Check sheet for the drawn part. Datum: minimum x, y, z corner. Units: mm. A direction names the side the tool comes from. Coordinates: 2 decimals unless noted, no trailing zeros. Order: outer loops, then holes, each group sorted by start corner. A loop starts at its lowest first (then second) coordinate and runs counter-clockwise, first axis right, second up.
1. Cross-section at D-D (y = 3.5). Enter the section's corners in (x, z), then the cut area to 3 significant figures.
2. Set-up check for the marked faces 1 and 2: record each of +Z, -Z, +X, -X, +Y, -Y from which the full face is reachable in a straight line by a thin tool's end or side.
3. Gauge pin test, flat ends, axial feed: pin 1 Ø4 at (x, y) = (9, 3) entering from +Z; pin 2 Ø2 at (y, z) = (7.5, 9) entering from -X; pin 3 Ø1 at (x, z) = (7.5, 14) entering from -Y; pin 4 Ø2 at (y, z) = (11, 12) entering from +X. Record the tip position at first contact, or that the pin passes through.
4. Draft check along Y on the marked faces 3, 4 and 5. Enter one of: released by +Y, released by -Y, zero draft, split by the parting line, or undercut.
5. Cross-section at A-A (z = 8). Enter the section's corners in (x, y).
6. Thickness scan on line 1 (X direction, y = 8, z = 9.25); line 2 (X direction, y = 8, z = 5); line 3 (Y direction, x = 5, z = 8). Record the ranges inside material, lowest first.
7. Cross-section at B-B (y = 7.75). Enter the section's corners in (x, z), then the cut area to 3 significant figures.
8. Cross-section at C-C (x = 5.5). Enter the section's corners in (y, z), then the cut area to 3 significant figures.
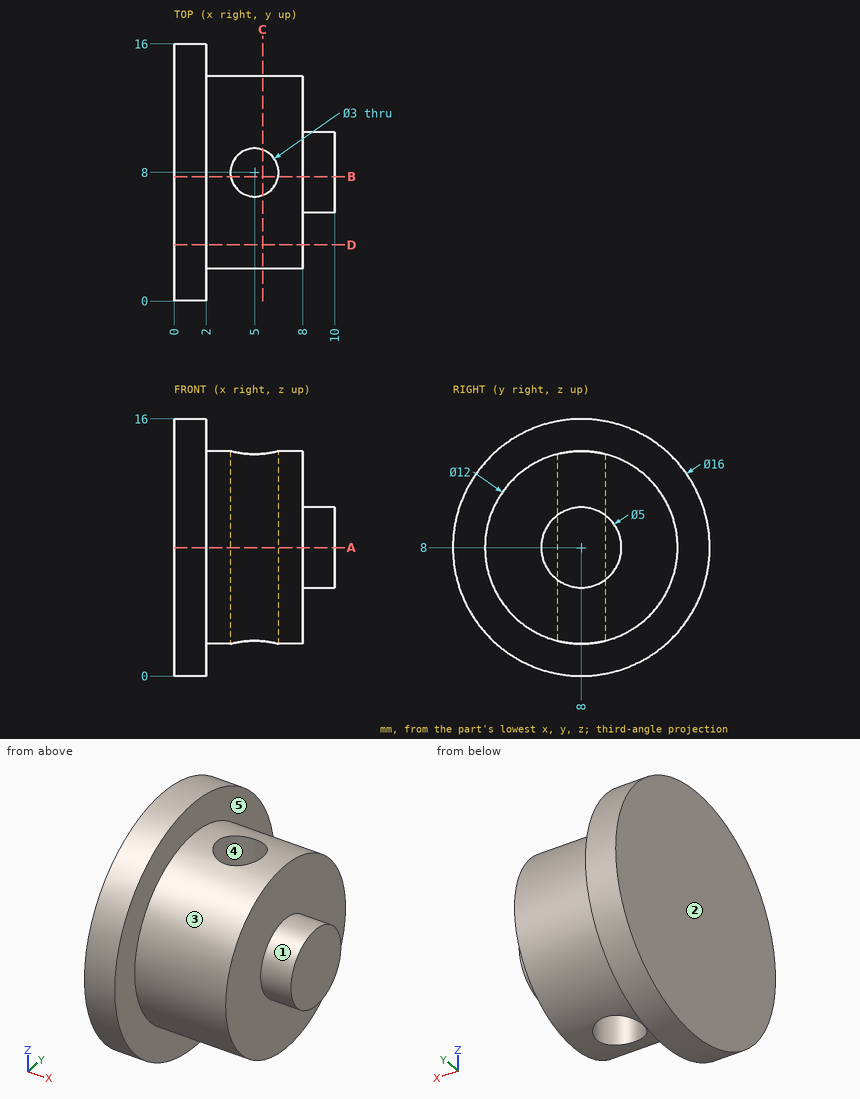
Data:
1. outline: (0, 1.39) - (2, 1.39) - (2, 4.03) - (8, 4.03) - (8, 11.97) - (2, 11.97) - (2, 14.61) - (0, 14.61) - close
1. area: 74.1 mm2
2. face 1: +X
2. face 2: +Z, -Z, -X, +Y, -Y
3. pin 1: stops at z = 13.03
3. pin 2: stops at x = 0
3. pin 3: stops at y = 5.6
3. pin 4: stops at x = 8
4. face 3: split by the parting line
4. face 4: undercut
4. face 5: zero draft
5. outline: (0, 0) - (2, 0) - (2, 2) - (8, 2) - (8, 5.5) - (10, 5.5) - (10, 10.5) - (8, 10.5) - (8, 14) - (2, 14) - (2, 16) - (0, 16) - close; hole circle Ø3 at (5, 8)
6. line 1: x = 0 to 3.5, 6.5 to 10
6. line 2: x = 0 to 3.5, 6.5 to 8
6. line 3: y = 2 to 6.5, 9.5 to 14
7. outline: (0, 0) - (2, 0) - (2, 2.01) - (3.52, 2.01) - (3.52, 13.99) - (2, 13.99) - (2, 16) - (0, 16) - close; (6.48, 2.01) - (8, 2.01) - (8, 5.51) - (10, 5.51) - (10, 10.49) - (8, 10.49) - (8, 13.99) - (6.48, 13.99) - close
7. area: 78.4 mm2
8. outline: (6.59, 2.17) - (6.59, 13.83) arc R6 ccw to start; (9.41, 2.17) arc R6 ccw to (9.41, 13.83) - close
8. area: 79.5 mm2
